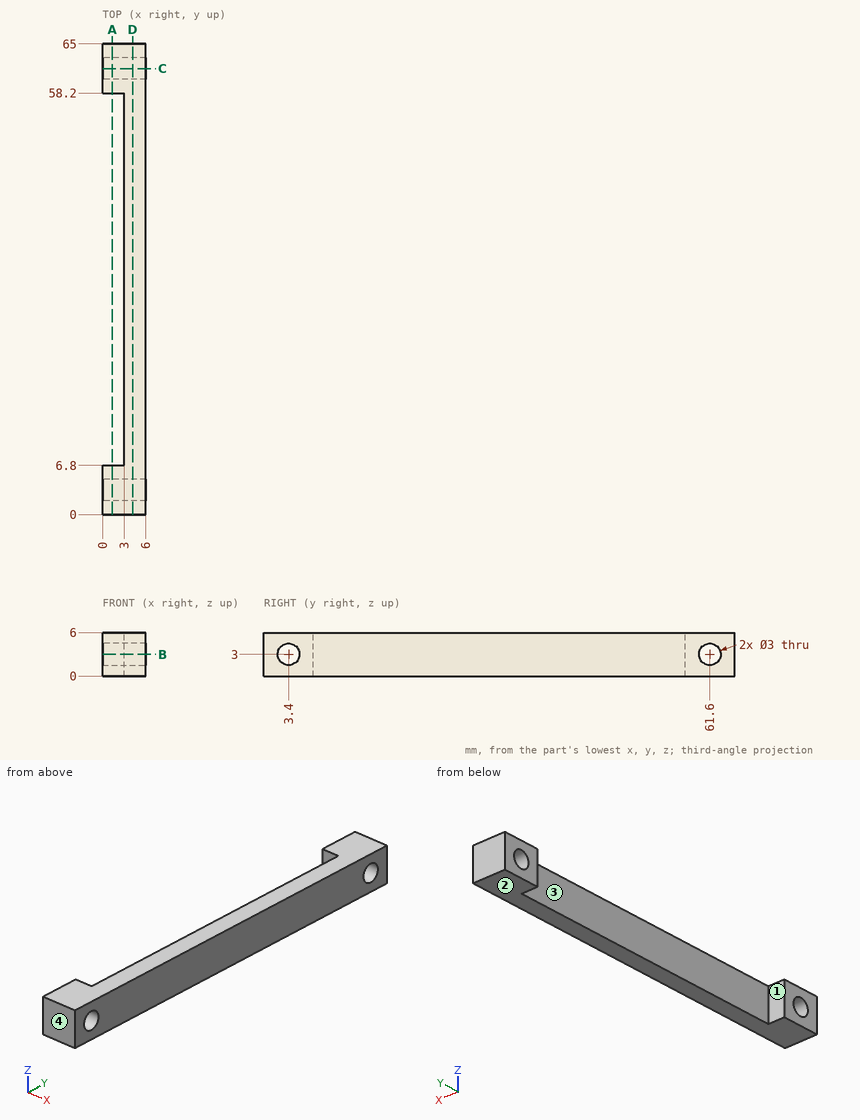
Study the drawing (mm; zero at the part's minimum x, y, z) and answer. Round coordinates to 2 decimals unless told otherwise and drop trailing zeros. Loops run counter-clockwise (first coordinate to the right, second up) from the corner with the lowest first, then second, coordinate; pieces in that order, holes last. Notation, with made-up numbers: (22.25, 46.5) - (48.25, 46.5) arc R13 ccw to (48.25, 68.5) - close; hole circle Ø11 at (59, 36). An arc over 180 degrees is marked (long way). Use one line per item in the form item = value. Start each with the question number.
1. Consider line 1 (Y direction, x = 3.75, z = 3); line 2 (Z direction, x = 1.3, y = 3.4); line 3 (Y direction, x = 2.25, z = 2.4). Determine where each line is inside the solid, lowest interval first. Write a range as [from, to].
2. The part is cut by section C-C on y = 61.6. Determine the outline of the cut face in (x, z).
3. For a pull along Y with two mould halves and no side action, classify the marked faces 1, 2, 3 and 4 as pulls with the +Y half, pulls with the -Y half, needs draft (parallel to the pull), parting line crosses it, or undercut.
4. The part is cut by section D-D on x = 4.15. Determine the outline of the cut face in (y, z), then the cut area to 3 significant figures.
5. The part is cut by section B-B on z = 3. Determine the outline of the cut face in (x, y).
6. Given pin 1 Ø3 at (y, z) = (23.5, 3) entering from -X, flat-ended and moving along its own axis, determine where the tip first touches the part or whether it passes through.
7. The part is cut by section A-A on x = 1.35. Determine the outline of the cut face in (y, z).
Geometry check:
q1.line_1 = [0, 1.9], [4.9, 60.1], [63.1, 65]
q1.line_2 = [0, 1.5], [4.5, 6]
q1.line_3 = [0, 2.03], [4.77, 6.8], [58.2, 60.23], [62.97, 65]
q2.outline = (0, 0) - (6, 0) - (6, 1.5) - (0, 1.5) - close; (0, 4.5) - (6, 4.5) - (6, 6) - (0, 6) - close
q3.face_1 = undercut
q3.face_2 = needs draft
q3.face_3 = undercut
q3.face_4 = pulls with the -Y half
q4.outline = (0, 0) - (65, 0) - (65, 6) - (0, 6) - close; hole circle Ø3 at (3.4, 3); hole circle Ø3 at (61.6, 3)
q4.area = 376 mm^2
q5.outline = (0, 0) - (6, 0) - (6, 1.9) - (0, 1.9) - close; (0, 4.9) - (6, 4.9) - (6, 60.1) - (0, 60.1) - (0, 58.2) - (3, 58.2) - (3, 6.8) - (0, 6.8) - close; (0, 63.1) - (6, 63.1) - (6, 65) - (0, 65) - close
q6.pin_1 = 3
q7.outline = (0, 0) - (6.8, 0) - (6.8, 6) - (0, 6) - close; (58.2, 0) - (65, 0) - (65, 6) - (58.2, 6) - close; hole circle Ø3 at (3.4, 3); hole circle Ø3 at (61.6, 3)
